Autodesk Inventor part; units mm, degrees
ref_plane "YZ Plane" through (0, 0, 0) normal (1, 0, 0) x (0, 1, 0)
ref_plane "XZ Plane" through (0, 0, 0) normal (0, 1, 0) x (-1, 0, 0)
ref_plane "XY Plane" through (0, 0, 0) normal (0, 0, 1) x (1, 0, 0)
sketch "Sketch1" plane through (0, 0, 0) normal (0, 1, 0) x (-1, 0, 0)
  arc A0 (38.1, 0) -> (-38.1, 0) centre (0, 0) ccw
  line L0 (38.1, 0) -> (38.1, -152.4)
  line L1 (-38.1, 0) -> (-38.1, -152.4)
  line L2 (0, -190.5) -> (0, 76.2)
  line L3 (53.34, 0) -> (-53.34, 0)
  line L4 (38.1, -152.4) -> (-38.1, -152.4)
  dimension "d0" = 76.2
  dimension "d1" = 152.4
  dimension "d2" = 152.4
extrude "Extrusion1" add sketch "Sketch1" along normal blind 15.875
sketch "Sketch2" plane through (0, 15.875, 0) normal (0, 1, 0) x (1, 0, 0)
  point P0 (0, 0)
  point P1 (0, 0)
hole "Hole1" at (0, 15.875, 0) direction (0, -1, 0) diameter 38.1 depth 15.875 tip angle 118
sketch "Sketch4" plane through (38.1, 0, 0) normal (1, 0, 0) x (0, 0, -1)
  line L0 (152.4, 15.875) -> (0, 15.875)
  line L1 (152.4, 15.875) -> (152.4, 50.8)
  line L2 (152.4, 50.8) -> (152.4, 88.9)
  line L3 (152.4, 88.9) -> (38.1, 88.9)
  line L4 (38.1, 88.9) -> (38.1, 15.875)
  line L5 (152.4, 50.8) -> (127, 88.9)
  line L6 (38.1, 50.8) -> (63.5, 88.9)
  line L7 (46.5667, 63.5) -> (143.9333, 63.5)
  point P0 (0, 0)
  dimension "d15" = 114.3
  dimension "d16" = 50.8
  dimension "d17" = 88.9
  dimension "d18" = 25.4
  dimension "d19" = 25.4
extrude "Extrusion2" add sketch "Sketch4" against normal blind 76.2 contours L0 L4 L6 L7 L5 L1
shell "Shell1" thickness 4.7625 removed faces 1 at (0, 0, -107.95)
sketch "Sketch5" plane through (38.1, 0, 0) normal (1, 0, 0) x (0, 0, -1)
  point P0 (0, 0)
sketch "Sketch6" plane through (38.1, 0, 0) normal (1, 0, 0) x (0, 0, -1)
  line L0 (38.1, 50.8) -> (38.1, 15.875)
  line L1 (38.1, 50.8) -> (38.1, 88.9)
  line L2 (38.1, 88.9) -> (152.4, 88.9)
  line L3 (152.4, 0) -> (152.4, 50.8)
  line L4 (152.4, 88.9) -> (152.4, 50.8)
  line L5 (46.5667, 63.5) -> (38.1, 50.8)
  line L6 (46.5667, 63.5) -> (63.5, 88.9)
  line L7 (152.4, 50.8) -> (143.9333, 63.5)
  line L8 (143.9333, 63.5) -> (127, 88.9)
  line L9 (46.5667, 63.5) -> (143.9333, 63.5)
  line L10 (0, 0) -> (152.4, 0)
  dimension "d23" = 38.1
extrude "Extrusion3" add sketch "Sketch6" against normal blind 76.2 contours L6 L2 L8 L9
sketch "Sketch8" plane through (38.1, 15.875, -38.1) normal (0, 0, 1) x (1, 0, 0)
  line L0 (-66.675, 47.625) -> (-9.525, 47.625)
  line L1 (0, 73.025) -> (-76.2, 73.025)
  line L2 (-66.675, 47.625) -> (-52.0103, 73.025)
  line L3 (-9.525, 47.625) -> (-24.1897, 73.025)
  line L4 (-52.0103, 73.025) -> (-24.1897, 73.025)
  point P0 (-38.1, -15.875)
  point P1 (-59.3427, 60.325)
  point P2 (-16.8573, 60.325)
  point P3 (-38.1, 73.025)
  point P4 (-38.1, 47.625)
  dimension "d31" = 57.15
  dimension "d32" = 25.4
  dimension "d33" = 60
extrude "Extrusion4" cut sketch "Sketch8" against normal blind 107.95
properties part number "Ch4 Part 4"
Work out the finished part from the listing and answer in its coordinate system (mm). A direction names the side the tool comes from. Coordinates: 2 decimals unless noted, no trailing zeros. Write each loop counter-clockwise with the first axis right and the second up, starting at its lowest first coordinate (ties: lowest second). Pieces come first, ordered by that corner, then holes. Notation, with made-up numbers: (48.5, 24) - (79.5, 24) arc R38 cw to (79.5, 62) - close; hole circle Ø1 at (-32.75, 69.5). An arc over 180 degrees is marked (long way). One line per question, with ' | ' between items.
1) For faces 1 (the face through (21.345, 76.022, -94.568)), 2 (the face through (-38.1, 35, -92)), 3 (the face through (-14, 11.112, -21)), 4 (the face through (1, 34, -38.1)), 5 (the face through (34, 0, -64)), determine the directions among +Z, -Z, +X, -X, +Y, -Y from which every point of the face is accessible in a straight line to the end or side of a thin tool.
Checks:
face 1: +Z, -Z | face 2: +Z, -Z, -X, +Y, -Y | face 3: -Y | face 4: +Z, +X, -X, +Y | face 5: +Z, -Z, +X, -X, -Y
2) The mould has two halves that part along Z. Classify faces 6 (the face through (-26, 88.9, -95)), 7 (the face through (0.84, 7.83, 38.09)), 8 (the face through (0.73, 5.48, 33.33)): +Z half, -Z half, draft (parallel to the pull), parting line (faces both ways), or undercut.
Checks:
face 6: draft | face 7: +Z half | face 8: undercut
3) Find section D-D, the plane x = -16. Determine the outline of the cut face in (y, z) (1 decimal).
Checks:
outline: (0, -152.4) - (50.8, -152.4) - (63.5, -143.9) - (63.5, -46.6) - (50.8, -38.1) - (15.9, -38.1) - (15.9, -10.3) - (0, -10.3) - (0, -17.6) - (11.1, -17.6) - (11.1, -42.9) - (49.4, -42.9) - (58.7, -49.1) - (58.7, -141.4) - (49.4, -147.6) - (0, -147.6) - close; (0, 10.3) - (15.9, 10.3) - (15.9, 34.6) - (0, 34.6) - (0, 29.2) - (11.1, 29.2) - (11.1, 17.6) - (0, 17.6) - close; (85.3, -129.4) - (88.9, -127) - (88.9, -63.5) - (85.3, -61.1) - close
4) Flat-ended cylindrical pins translate along their axes: P1, Ø1, axis at x = 29.5, y = 16, coming from the +Z side; P2, Ø2, axis at x = -23.5, y = 63, coming from the +Z side; P3, Ø3, axis at x = 0.5, z = -91, coming from the +Y side; P4, Ø3, axis at y = 18.5, z = -31.5, coming from the -X side. Find the tip coordinate at first contact, or state that the pin passes through.
Checks:
P1: z = 24.69 | P2: z = -45.57 | P3: y = 63.5 | P4: through
5) Find section A-A, the plane y = 8.5. Give the number of separate pieces and of enclosed holes in the cut face, and give its area (3 significant figures).
Checks:
separate pieces: 2 | enclosed holes: 2 | area: 2,940 mm2
6) Consider probe 1 along X at (y, z) = (10, 0); probe 2 along Z at (x, y) = (0, 6); probe 3 along Z at (x, y) = (5, 21). Determine where each line is inside the solid, lowest interval first. Write a range as [from, to].
Checks:
probe 1: [-38.1, -33.34], [-23.81, -19.05], [19.05, 23.81], [33.34, 38.1] | probe 2: [-152.4, -147.64], [-23.81, -19.05], [19.05, 23.81], [33.34, 38.1] | probe 3: [-152.4, -147.64], [-42.86, -38.1]
7) Find section C-C, the plane z = 5. Determine the outline of the cut face in (x, y) (1 decimal), and give its area (3 significant figures).
Checks:
outline: (-37.8, 0) - (-33, 0) - (-33, 11.1) - (-23.3, 11.1) - (-23.3, 0) - (-18.4, 0) - (-18.4, 15.9) - (-37.8, 15.9) - close; (18.4, 0) - (23.3, 0) - (23.3, 11.1) - (33, 11.1) - (33, 0) - (37.8, 0) - (37.8, 15.9) - (18.4, 15.9) - close | area: 400 mm2
